from build123d import *

# Parameters (mm, degrees)
SKETCH_1_R               = 15
SKETCH_1_R_2             = 5
EXTRUDE_4_DEPTH          = 3
SKETCH_1_R_3             = 3.5
SKETCH_1_R_4             = 2.1
EXTRUDE_4_2_DEPTH        = 3
EXTRUDE_5_DEPTH          = 3
PATTERN_CIRCULAR_2_COUNT = 4
SKETCH_6_R               = 3.5
SKETCH_6_R_2             = 2.1
EXTRUDE_6_DEPTH          = 3
PATTERN_CIRCULAR_3_COUNT = 4
SKETCH_7_R               = 15
SKETCH_7_R_2             = 5
EXTRUDE_7_DEPTH          = 46
CUT_EXTRUDE_1_DEPTH      = 46
PATTERN_CIRCULAR_4_COUNT = 4
SKETCH_11_R              = 1.5
CUT_EXTRUDE_2_DEPTH      = 3
PATTERN_CIRCULAR_5_COUNT = 4
EXTRUDE_8_DEPTH          = 3
EXTRUDE_9_DEPTH          = 3
EXTRUDE_10_DEPTH         = 3
EXTRUDE_11_DEPTH         = 3
EXTRUDE_13_DEPTH         = 3
EXTRUDE_14_DEPTH         = 3
CUT_EXTRUDE_3_DEPTH      = 2.5
SKETCH_19_R              = 1.5
CUT_EXTRUDE_4_DEPTH      = 2.5
SKETCH_20_R              = 1.5
CUT_EXTRUDE_5_DEPTH      = 2.5
SKETCH_21_R              = 15
SKETCH_21_R_2            = 5
EXTRUDE_15_DEPTH         = 3
SKETCH_22_R              = 1.5
CUT_EXTRUDE_6_DEPTH      = 3
PATTERN_CIRCULAR_6_COUNT = 4
EXTRUDE_16_DEPTH         = 3
CUT_EXTRUDE_7_DEPTH      = 3
SKETCH_25_R              = 15
SKETCH_25_R_2            = 5
EXTRUDE_17_DEPTH         = 43
SKETCH_27_R              = 1.5
CUT_EXTRUDE_8_DEPTH      = 46
SKETCH_28_R              = 2.75
CUT_EXTRUDE_9_DEPTH      = 43
SKETCH_29_R              = 1.5
CUT_EXTRUDE_10_DEPTH     = 46
PATTERN_CIRCULAR_7_COUNT = 4
CUT_EXTRUDE_11_DEPTH     = 43
PATTERN_CIRCULAR_8_COUNT = 4
SKETCH_31_R              = 26.244176336
CUT_EXTRUDE_12_DEPTH     = 100


with BuildPart() as part:
    # Sketch 1 → Extrude 4 (new body)
    with BuildSketch(Plane(origin=(0, 0, 0), x_dir=(1, 0, 0), z_dir=(0, 1, 0))):
        with Locations((-5.372895461, -8.931727747)):
            Circle(SKETCH_1_R)
        with Locations((-5.372895461, -8.931727747)):
            Circle(SKETCH_1_R_2, mode=Mode.SUBTRACT)
    extrude(amount=EXTRUDE_4_DEPTH)



with BuildPart() as body_2:
    # Sketch 1 → Extrude 4 2 (new body)
    with BuildSketch(Plane(origin=(0, 0, 0), x_dir=(1, 0, 0), z_dir=(0, 1, 0))):
        with Locations((-22.372895461, 8.068272253)):
            Circle(SKETCH_1_R_3)
        with Locations((-22.372895461, 8.068272253)):
            Circle(SKETCH_1_R_4, mode=Mode.SUBTRACT)
    extrude(amount=EXTRUDE_4_2_DEPTH)


with BuildPart() as part_1:
    add(part.part)

    add(body_2.part)  # Extrude 5 merges body 2
    # Sketch 5 → Extrude 5 (add)
    with BuildSketch(Plane(origin=(0, 0, 0), x_dir=(1, 0, 0), z_dir=(0, 1, 0))):
        Polygon((-22.372895461, 4.568272253), (-10.372895461, -8.931727747), (-10.372895461, -3.931727747), (-5.372895461, -3.931727747), (-18.872895461, 8.068272253), align=None)
    extrude_5 = extrude(amount=EXTRUDE_5_DEPTH)

    # Pattern Circular 2: Extrude 5 ×4 about axis
    pattern_circular_2_axis = Axis((-5.372895461, 0, 8.931727747), (0, 1, 0))
    for i in range(1, PATTERN_CIRCULAR_2_COUNT):
        add(extrude_5.rotate(pattern_circular_2_axis, i * 360 / PATTERN_CIRCULAR_2_COUNT))

    # Sketch 6 → Extrude 6 (add)
    with BuildSketch(Plane(origin=(0, 3, 0), x_dir=(1, 0, 0), z_dir=(0, 1, 0))):
        with Locations((11.627104539, 8.068272253)):
            Circle(SKETCH_6_R)
        with Locations((11.627104539, 8.068272253)):
            Circle(SKETCH_6_R_2, mode=Mode.SUBTRACT)
    extrude_6 = extrude(amount=-EXTRUDE_6_DEPTH)

    # Pattern Circular 3: Extrude 6 ×4 about axis
    pattern_circular_3_axis = Axis((-5.372895461, 0, 8.931727747), (0, 1, 0))
    for i in range(1, PATTERN_CIRCULAR_3_COUNT):
        add(extrude_6.rotate(pattern_circular_3_axis, i * 360 / PATTERN_CIRCULAR_3_COUNT))

    # Sketch 7 → Extrude 7 (add)
    with BuildSketch(Plane.XZ):
        with Locations((-5.372895461, 8.931727747)):
            Circle(SKETCH_7_R)
        with Locations((-5.372895461, 8.931727747)):
            Circle(SKETCH_7_R_2, mode=Mode.SUBTRACT)
    extrude(amount=EXTRUDE_7_DEPTH)

    # Sketch 9 → Cut-Extrude 1 (cut)
    with BuildSketch(Plane(origin=(0, 3, 0), x_dir=(1, 0, 0), z_dir=(0, 1, 0))):
        Polygon((0.876311502, -19.070022006), (-1.369054096, -16.824656408), (-0.547193246, -13.757429961), (2.520033201, -12.935569112), (4.765398798, -15.180934709), (3.943537949, -18.248161156), align=None)
    cut_extrude_1 = extrude(amount=-CUT_EXTRUDE_1_DEPTH, mode=Mode.SUBTRACT)

    # Pattern Circular 4: Cut-Extrude 1 ×4 about axis
    pattern_circular_4_axis = Axis((-5.372895461, 0, 8.931727747), (0, 1, 0))
    for i in range(1, PATTERN_CIRCULAR_4_COUNT):
        add(cut_extrude_1.rotate(pattern_circular_4_axis, i * 360 / PATTERN_CIRCULAR_4_COUNT), mode=Mode.SUBTRACT)

    # Sketch 11 → Cut-Extrude 2 (cut)
    with BuildSketch(Plane(origin=(0, -43, 0), x_dir=(1, 0, 0), z_dir=(0, 1, 0))):
        with Locations((1.698172351, -1.860659935)):
            Circle(SKETCH_11_R)
    cut_extrude_2 = extrude(amount=-CUT_EXTRUDE_2_DEPTH, mode=Mode.SUBTRACT)

    # Pattern Circular 5: Cut-Extrude 2 ×4 about axis
    pattern_circular_5_axis = Axis((-5.372895461, 0, 8.931727747), (0, 1, 0))
    for i in range(1, PATTERN_CIRCULAR_5_COUNT):
        add(cut_extrude_2.rotate(pattern_circular_5_axis, i * 360 / PATTERN_CIRCULAR_5_COUNT), mode=Mode.SUBTRACT)

    # Sketch 12 → Extrude 8 (add)
    with BuildSketch(Plane(origin=(0, 3, 0), x_dir=(1, 0, 0), z_dir=(0, 1, 0))):
        Polygon((15.127104539, 8.068272253), (15.127104539, -25.931727747), (11.627104539, -22.431727747), (11.627104539, 4.568272253), align=None)
    extrude(amount=-EXTRUDE_8_DEPTH)

    # Sketch 13 → Extrude 9 (add)
    with BuildSketch(Plane(origin=(0, 3, 0), x_dir=(1, 0, 0), z_dir=(0, 1, 0))):
        Polygon((11.627104539, 11.568272253), (-22.372895461, 11.568272253), (-18.872895461, 8.068272253), (8.127104539, 8.068272253), align=None)
    extrude(amount=-EXTRUDE_9_DEPTH)

    # Sketch 14 → Extrude 10 (add)
    with BuildSketch(Plane(origin=(0, 3, 0), x_dir=(1, 0, 0), z_dir=(0, 1, 0))):
        Polygon((-25.872895461, 8.068272253), (-25.872895461, -25.931727747), (-22.372895461, -22.431727747), (-22.372895461, 4.568272253), align=None)
    extrude(amount=-EXTRUDE_10_DEPTH)

    # Sketch 15 → Extrude 11 (add)
    with BuildSketch(Plane(origin=(0, 3, 0), x_dir=(1, 0, 0), z_dir=(0, 1, 0))):
        Polygon((-22.372895461, -29.431727747), (11.627104539, -29.431727747), (8.127104539, -25.931727747), (-18.872895461, -25.931727747), align=None)
    extrude(amount=-EXTRUDE_11_DEPTH)

    # Sketch 16 → Extrude 13 (add)
    with BuildSketch(Plane.XZ):
        Polygon((-10.747895461, -4.193272253), (0.002104539, -4.193272253), (5.163560245, -8.068272253), (4.99115505, -11.568272253), (0.002104539, -14.943272253), (-10.747895461, -14.943272253), (-15.736945971, -11.568272253), (-15.909351166, -8.068272253), align=None)
        Polygon((-7.57246898, -9.568272253), (-9.16018222, -6.818272253), (-12.335608701, -6.818272253), (-13.923321941, -9.568272253), (-12.335608701, -12.318272253), (-9.16018222, -12.318272253), align=None, mode=Mode.SUBTRACT)
        Polygon((3.17753102, -9.568272253), (1.58981778, -6.818272253), (-1.585608701, -6.818272253), (-3.173321941, -9.568272253), (-1.585608701, -12.318272253), (1.58981778, -12.318272253), align=None, mode=Mode.SUBTRACT)
    extrude(amount=-EXTRUDE_13_DEPTH)

    # Sketch 18 → Extrude 14 (add)
    with BuildSketch(Plane.XZ):
        Polygon((-7.57246898, -9.568272253), (-9.16018222, -6.818272253), (-12.335608701, -6.818272253), (-13.923321941, -9.568272253), (-12.335608701, -12.318272253), (-9.16018222, -12.318272253), align=None)
        Polygon((3.17753102, -9.568272253), (1.58981778, -6.818272253), (-1.585608701, -6.818272253), (-3.173321941, -9.568272253), (-1.585608701, -12.318272253), (1.58981778, -12.318272253), align=None)
    extrude(amount=-EXTRUDE_14_DEPTH)

    # Sketch 17 → Cut-Extrude 3 (cut)
    with BuildSketch(Plane.XZ):
        Polygon((-7.57246898, -9.568272253), (-9.16018222, -6.818272253), (-12.335608701, -6.818272253), (-13.923321941, -9.568272253), (-12.335608701, -12.318272253), (-9.16018222, -12.318272253), align=None)
        Polygon((3.17753102, -9.568272253), (1.58981778, -6.818272253), (-1.585608701, -6.818272253), (-3.173321941, -9.568272253), (-1.585608701, -12.318272253), (1.58981778, -12.318272253), align=None)
    extrude(amount=-CUT_EXTRUDE_3_DEPTH, mode=Mode.SUBTRACT)

    # Sketch 19 → Cut-Extrude 4 (cut)
    with BuildSketch(Plane.XZ.offset(-2.5)):
        with Locations((0.002104539, -9.568272253)):
            Circle(SKETCH_19_R)
    extrude(amount=-CUT_EXTRUDE_4_DEPTH, mode=Mode.SUBTRACT)

    # Sketch 20 → Cut-Extrude 5 (cut)
    with BuildSketch(Plane.XZ.offset(-2.5)):
        with Locations((-10.747895461, -9.568272253)):
            Circle(SKETCH_20_R)
    extrude(amount=-CUT_EXTRUDE_5_DEPTH, mode=Mode.SUBTRACT)

    # Sketch 8 → Extrude 16 (add)
    with BuildSketch(Plane.XZ.offset(46)):
        Polygon((3.943537949, 18.248161156), (0.876311502, 19.070022006), (-1.369054096, 16.824656408), (-0.547193246, 13.757429961), (2.520033201, 12.935569112), (4.765398798, 15.180934709), align=None)
    extrude(amount=EXTRUDE_16_DEPTH)

    # Sketch 24 → Cut-Extrude 7 (cut)
    with BuildSketch(Plane.XZ.offset(49)):
        Polygon((4.765398798, 15.180934709), (3.943537949, 18.248161156), (0.876311502, 19.070022006), (-1.369054096, 16.824656408), (-0.547193246, 13.757429961), (2.520033201, 12.935569112), align=None)
    extrude(amount=-CUT_EXTRUDE_7_DEPTH, mode=Mode.SUBTRACT)


with BuildPart() as body_2_2:
    # Sketch 21 → Extrude 15 (new body)
    with BuildSketch(Plane(origin=(0, 0, 0), x_dir=(1, 0, 0), z_dir=(0, 1, 0))):
        with Locations((59.665545214, -8.931727747)):
            Circle(SKETCH_21_R)
        with Locations((59.665545214, -8.931727747)):
            Circle(SKETCH_21_R_2, mode=Mode.SUBTRACT)
    extrude(amount=EXTRUDE_15_DEPTH)

    # Sketch 22 → Cut-Extrude 6 (cut)
    with BuildSketch(Plane.XZ):
        with Locations((59.665545214, 18.931727747)):
            Circle(SKETCH_22_R)
    cut_extrude_6 = extrude(amount=-CUT_EXTRUDE_6_DEPTH, mode=Mode.SUBTRACT)

    # Pattern Circular 6: Cut-Extrude 6 ×4 about axis
    pattern_circular_6_axis = Axis((59.665545214, 0, 8.931727747), (0, 1, 0))
    for i in range(1, PATTERN_CIRCULAR_6_COUNT):
        add(cut_extrude_6.rotate(pattern_circular_6_axis, i * 360 / PATTERN_CIRCULAR_6_COUNT), mode=Mode.SUBTRACT)

    # Sketch 25 → Extrude 17 (add)
    with BuildSketch(Plane.XZ):
        with Locations((59.665545214, 8.931727747)):
            Circle(SKETCH_25_R)
        with Locations((59.665545214, 8.931727747)):
            Circle(SKETCH_25_R_2, mode=Mode.SUBTRACT)
    extrude(amount=EXTRUDE_17_DEPTH)

    # Sketch 27 → Cut-Extrude 8 (cut)
    with BuildSketch(Plane(origin=(0, 3, 0), x_dir=(1, 0, 0), z_dir=(0, 1, 0))):
        with Locations((59.665545214, 1.068272253)):
            Circle(SKETCH_27_R)
        with Locations((69.665545214, -8.931727747)):
            Circle(SKETCH_27_R)
        with Locations((59.665545214, -18.931727747)):
            Circle(SKETCH_27_R)
        with Locations((49.665545214, -8.931727747)):
            Circle(SKETCH_27_R)
    extrude(amount=-CUT_EXTRUDE_8_DEPTH, mode=Mode.SUBTRACT)

    # Sketch 28 → Cut-Extrude 9 (cut)
    with BuildSketch(Plane.XZ.offset(43)):
        with Locations((59.665545214, 18.931727747)):
            Circle(SKETCH_28_R)
        with Locations((49.665545214, 8.931727747)):
            Circle(SKETCH_28_R)
        with Locations((59.665545214, -1.068272253)):
            Circle(SKETCH_28_R)
        with Locations((69.665545214, 8.931727747)):
            Circle(SKETCH_28_R)
    extrude(amount=-CUT_EXTRUDE_9_DEPTH, mode=Mode.SUBTRACT)

    # Sketch 29 → Cut-Extrude 10 (cut)
    with BuildSketch(Plane(origin=(0, 3, 0), x_dir=(1, 0, 0), z_dir=(0, 1, 0))):
        with Locations((66.736613026, -1.860659935)):
            Circle(SKETCH_29_R)
    cut_extrude_10 = extrude(amount=-CUT_EXTRUDE_10_DEPTH, mode=Mode.SUBTRACT)

    # Pattern Circular 7: Cut-Extrude 10 ×4 about axis
    pattern_circular_7_axis = Axis((59.665545214, 0, 8.931727747), (0, 1, 0))
    for i in range(1, PATTERN_CIRCULAR_7_COUNT):
        add(cut_extrude_10.rotate(pattern_circular_7_axis, i * 360 / PATTERN_CIRCULAR_7_COUNT), mode=Mode.SUBTRACT)

    # Sketch 30 → Cut-Extrude 11 (cut)
    with BuildSketch(Plane(origin=(0, 3, 0), x_dir=(1, 0, 0), z_dir=(0, 1, 0))):
        Polygon((64.491247429, -4.106025533), (67.558473876, -4.927886382), (69.803839473, -2.682520785), (68.981978624, 0.384705662), (65.914752177, 1.206566512), (63.669386579, -1.038799086), align=None)
    cut_extrude_11 = extrude(amount=-CUT_EXTRUDE_11_DEPTH, mode=Mode.SUBTRACT)

    # Pattern Circular 8: Cut-Extrude 11 ×4 about axis
    pattern_circular_8_axis = Axis((59.665545214, 0, 8.931727747), (0, 1, 0))
    for i in range(1, PATTERN_CIRCULAR_8_COUNT):
        add(cut_extrude_11.rotate(pattern_circular_8_axis, i * 360 / PATTERN_CIRCULAR_8_COUNT), mode=Mode.SUBTRACT)

    # Sketch 31 → Cut-Extrude 12 (cut)
    with BuildSketch(Plane(origin=(0, 3, 0), x_dir=(1, 0, 0), z_dir=(0, 1, 0))):
        with Locations((59.665545214, -8.931727747)):
            Circle(SKETCH_31_R)
    extrude(amount=-CUT_EXTRUDE_12_DEPTH, mode=Mode.SUBTRACT)


solid = part_1.part
Can you work these out from the model? Positions are in its coordinate system, mm. A direction names the side the tool comes from. Coordinates: 2 decimals unless noted, no trailing zeros. Order: outer loops, then holes, each group sorted by start corner. A loop starts at its lowest first (then second) coordinate and runs counter-clockwise, first axis right, second up. Notation, with made-up numbers: M 1,1.5 L 59,1.5 A30 ccw 59,33.5 Z; hole C -30.5,27 d6. An arc over 180 degrees is marked long. Write item = value, one per line.
(1) I need wall thicknesses on line 1 along Z through (x, y) = (-5.5, -19); line 2 along Z through (x, y) = (-13.5, -27.5); line 3 along X through (y, z) = (-32, 15.5). Which ranges of each line are inside material? Lowest first, please. Write a range as [from, to].
Results are:
line_1 = [-6.07, 3.93], [13.93, 23.93]
line_2 = [-3.68, -0.7], [4.69, 13.17], [18.57, 21.54]
line_3 = [-18.86, -15.43], [-9.73, -1.01], [4.68, 8.11]
(2) Suppose I cut it at A-A on x = -5.5. Please give me the cut outline in (y, z).
Results are:
outline = M -46,-6.07 L 0,-6.07 L 0,-14.94 L 3,-14.94 L 3,3.93 L -46,3.93 Z; M -46,13.93 L 3,13.93 L 3,23.93 L -46,23.93 Z; M 0,25.93 L 3,25.93 L 3,29.43 L 0,29.43 Z
(3) Suppose I cut it at C-C on y = -32. Please give me the cut outline in (x, z), plus the area to 3 significant figures.
Results are:
outline = C -5.37,8.93 d30; hole M -15.51,2.68 L -14.69,-0.38 L -11.62,-1.21 L -9.38,1.04 L -10.2,4.11 L -13.27,4.93 Z; hole M -15.51,15.18 L -13.27,12.94 L -10.2,13.76 L -9.38,16.82 L -11.62,19.07 L -14.69,18.25 Z; hole C -5.37,8.93 d10; hole M -1.37,1.04 L 0.88,-1.21 L 3.94,-0.38 L 4.77,2.68 L 2.52,4.93 L -0.55,4.11 Z; hole M -1.37,16.82 L -0.55,13.76 L 2.52,12.94 L 4.77,15.18 L 3.94,18.25 L 0.88,19.07 Z
area = 524 mm2
(4) For faces 1 (the face through (-15.095, -19.678, 16.736)), 2 (the face through (-2.391, 1.232, -10.924)), 3 (the face through (-5, 2, 25.932)), 4 (the face through (-10.2, 3, 6.9)), which set-ups out of +Z, -Z, +X, -X, +Y, -Y let a thin tool reach every point of the face, with its end or its side?
Results are:
face_1 = +Y
face_2 = -Y
face_3 = +Y, -Y
face_4 = +Z, -Z, +X, -X, +Y
(5) Suppose I cut it at D-D on z = 12. Please give me the cut outline in (x, y).
Results are:
outline = M -25.87,0 L -22.37,0 L -22.37,3 L -25.87,3 Z; M -20.06,-46 L -9.32,-46 L -9.32,3 L -20.06,3 Z; M -1.43,-46 L 9.31,-46 L 9.31,3 L -1.43,3 Z; M 11.63,0 L 15.13,0 L 15.13,3 L 11.63,3 Z
(6) For pin 1 Ø3.5 at (x, z) = (0, -9.57) entering from -Y; pin 2 Ø5 at (x, z) = (-13, 16) entering from -Y; pin 3 Ø3 at (x, z) = (1.5, 1.5) entering from +Y; pin 4 Ø8 at (y, z) = (-28.5, 24.5) entering from -X, each with a flat end and sliding along its axis, tell me the tip position at first contact or that it passes through.
Results are:
pin_1 = 2.5
pin_2 = -46
pin_3 = -43
pin_4 = -14.92
(7) Suppose I cut it at B-B on z = 25. Please give me the cut outline in (x, y), plus the area to 3 significant figures.
Results are:
outline = M -25.87,0 L -24.25,0 L -24.25,3 L -25.87,3 Z; M -20.49,0 L -17.82,0 L -17.82,3 L -20.49,3 Z; M 7.08,0 L 9.75,0 L 9.75,3 L 7.08,3 Z; M 13.51,0 L 15.13,0 L 15.13,3 L 13.51,3 Z
area = 25.7 mm2
(8) If we mould it in two halves opening along X, with no side actions, what happens to faces 5 (the face through (-14.4, -19.68, 14.07)), 6 (the face through (-19, 2, -11.568))? For each: pulls with the +X half, pulls with the -X half, needs draft (parallel to the pull), parting line crosses it, or undercut.
Results are:
face_5 = undercut
face_6 = needs draft
